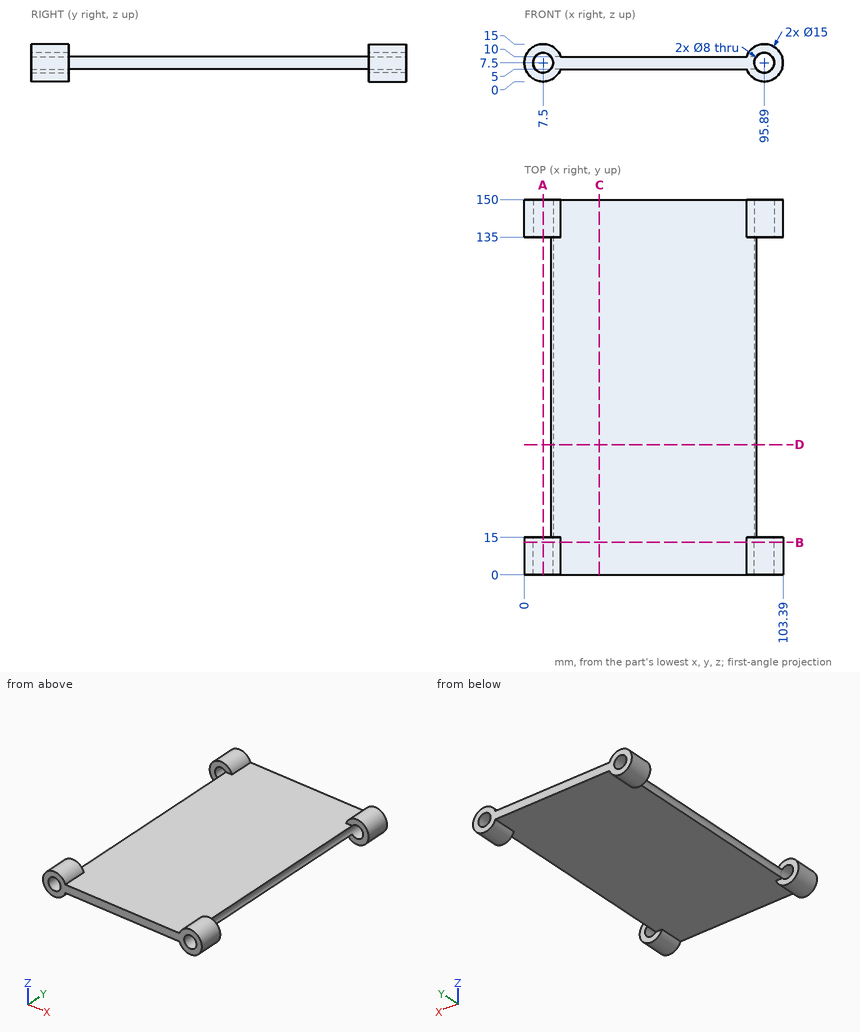
Print and shaded views of the part. All mm, measured from the part's lowest x, y and z. Coordinates: 2 decimals unless noted, no trailing zeros. Write each loop counter-clockwise with the first axis right and the second up, starting at its lowest first coordinate (ties: lowest second). Pieces come first, ordered by that corner, then holes.
(1) Cut at D-D, the plane y = 52. List the corners of the cut face in (x, z).
(2) Cut at B-B, the plane y = 13. List the corners of the cut face in (x, z), and give its area (3 significant figures).
(3) Flat gauge pins, fed straight in: pin 1 (5 mm diameter, centred on x = 53.5, z = 13, fed in from -Y); pin 2 (1 mm diameter, centred on y = 61.5, z = 6.5, fed in from -X); pin 3 (4 mm diameter, centred on x = 66.5, y = 45, fed in from -Z); pin 4 (24.5 mm diameter, centred on x = 54.5, y = 83, fed in from +Z). Where does each tip first touch, or does it go through?
(4) Cut at A-A, the plane x = 7.5. List the corners of the cut face in (y, z), and give its area (3 significant figures).
(5) Drill centre lines: probe 1 along X at (y, z) = (6, 7.5); probe 2 along Z at (x, y) = (95.89, 8.5); probe 3 along X at (y, z) = (82.5, 8). Where is each one in solid material? Low to high.
(6) Cut at C-C, the plane x = 30. List the corners of the cut face in (y, z).
Geometry says:
1. outline: (10.62, 5) - (92.77, 5) arc R4 cw to (92.77, 10) - (10.62, 10) arc R4 cw to start
2. outline: (14.57, 5) - (88.82, 5) arc R7.5 ccw (long way) to (88.82, 10) - (14.57, 10) arc R7.5 ccw (long way) to start; hole circle Ø8 at (7.5, 7.5); hole circle Ø8 at (95.89, 7.5)
2. area: 621 mm2
3. pin 1: passes through
3. pin 2: stops at x = 11.21
3. pin 3: stops at z = 5
3. pin 4: stops at z = 10
4. outline: (0, 0) - (15, 0) - (15, 3.5) - (0, 3.5) - close; (0, 11.5) - (15, 11.5) - (15, 15) - (0, 15) - close; (135, 0) - (150, 0) - (150, 3.5) - (135, 3.5) - close; (135, 11.5) - (150, 11.5) - (150, 15) - (135, 15) - close
4. area: 210 mm2
5. probe 1: x = 0 to 3.5, 11.5 to 91.89, 99.89 to 103.39
5. probe 2: z = 0 to 3.5, 11.5 to 15
5. probe 3: x = 11.47 to 91.92
6. outline: (0, 5) - (150, 5) - (150, 10) - (0, 10) - close
